from build123d import *

# Parameters (mm, degrees)
F1_DEPTH = 51.5
F2_W     = 13
F2_H     = 22.75
F3_DEPTH = 13
F4_W     = 13
F4_H     = 3
F5_DEPTH = 5


with BuildPart() as f1:
    # F0 (on Top) → F1 (new body)
    with BuildSketch(Plane.XY):
        Polygon((-10.25, 26.798756), (-29.50686, 0), (-5, 0), (-5, 8.67), (5, 8.67), (5, 0), (29.50686, 0), (10.25, 26.798756), align=None)
    extrude(amount=F1_DEPTH)

    # F2 (on face) → F3 (cut)
    with BuildSketch(Plane.XY.offset(51.5)):
        with Locations((0, 15.423756)):
            Rectangle(F2_W, F2_H)
    extrude(amount=-F3_DEPTH, mode=Mode.SUBTRACT)

    # F4 (on face) → F5 (cut)
    with BuildSketch(Plane.XY.offset(38.5)):
        with Locations((0, 23.298756)):
            Rectangle(F4_W, F4_H)
    extrude(amount=-F5_DEPTH, mode=Mode.SUBTRACT)


solid = f1.part
CAD build for the part. Positions are in the model's coordinates, mm. A direction names the side the tool comes from. Give positions to 0.01 mm unless a question says otherwise; leave off trailing zeros. Write each loop counter-clockwise with the first axis right and the second up, starting at its lowest first coordinate (ties: lowest second). Pieces come first, ordered by that corner, then holes. Notation, with made-up numbers: M 13.25,47.25 L 63.25,47.25 A32 cw 63.25,81.25 Z; hole C -34.5,64.5 d2. An arc over 180 degrees is marked long. Put each result on its own line as item: value. Start each with the question number.
(1) Band-saw the part on D-D, the plane y = 13.25. Write the cut outline in (x, z), and give its area (3 significant figures).
(2) Probe L1, parallel to Y at x = 4, z = 25.5; L2, parallel to X at y = 4, z = 18.5; L3, parallel to X at y = 15, z = 42. List the from-to ranges inside material, lowest first.
(3) Which spindle directions (+Z, -Z, +X, -X, +Y, -Y) get a long thin tool onto all of the face, cutting with end or side? Do faces 4 (the face through (-17, 0, 25)), 5 (the face through (0, 15, 38.5)), 6 (the face through (14, 11, 51.5)), 7 (the face through (-5, 4, 25)), 8 (the face through (0, 24.799, 36)). Say none if no direction does.
(4) Flat gauge pins, fed straight in: pin 1 Ø2 at (x, y) = (-3, 14.5) entering from +Z; pin 2 Ø5.5 at (y, z) = (10.5, 41.5) entering from -X; pin 3 Ø2.5 at (x, z) = (-0.5, 37) entering from -Y; pin 4 Ø1.5 at (x, y) = (15.5, 21) entering from -Z. Where does each tip first touch, or does it go through?
(5) Band-saw the part on C-C, the plane z = 37. Write the cut outline in (x, y).
(6) Mould opens along X. For faces 1 (the face through (0, 26.799, 25)), 2 (the face through (0, 21.799, 36)), 3 (the face through (-19.74, 13.59, 25.39)) say: +X half, -X half, draft (parallel to the pull), parting line (faces both ways), or undercut.
(7) Band-saw the part on B-B, the plane x = -0.5. Write the cut outline in (y, z).
(8) Band-saw the part on A-A, the plane z = 44. Write the cut outline in (x, y), and give its area (3 significant figures).
Response values:
1. outline: M -19.99,0 L 19.99,0 L 19.99,51.5 L 6.5,51.5 L 6.5,38.5 L -6.5,38.5 L -6.5,51.5 L -19.99,51.5 Z
1. area: 1,890 mm2
2. L1: y = 8.67 to 26.8
2. L2: x = -26.63 to -5, 5 to 26.63
2. L3: x = -18.73 to -6.5, 6.5 to 18.73
3. face 4: +Z, -Z, +X, -X, -Y
3. face 5: +Z, +Y
3. face 6: +Z, +X, -X, +Y, -Y
3. face 7: +Z, -Z, -Y
3. face 8: +Z
4. pin 1: stops at z = 38.5
4. pin 2: stops at x = -23.94
4. pin 3: stops at y = 8.67
4. pin 4: passes through
5. outline: M -29.51,0 L -5,0 L -5,8.67 L 5,8.67 L 5,0 L 29.51,0 L 10.25,26.8 L -10.25,26.8 Z; hole M -6.5,21.8 L 6.5,21.8 L 6.5,24.8 L -6.5,24.8 Z
6. face 1: draft
6. face 2: undercut
6. face 3: -X half
7. outline: M 8.67,0 L 26.8,0 L 26.8,38.5 L 24.8,38.5 L 24.8,33.5 L 21.8,33.5 L 21.8,38.5 L 8.67,38.5 Z
8. outline: M -29.51,0 L -5,0 L -5,4.05 L -6.5,4.05 L -6.5,26.8 L -10.25,26.8 Z; M 5,0 L 29.51,0 L 10.25,26.8 L 6.5,26.8 L 6.5,4.05 L 5,4.05 Z
8. area: 729 mm2
